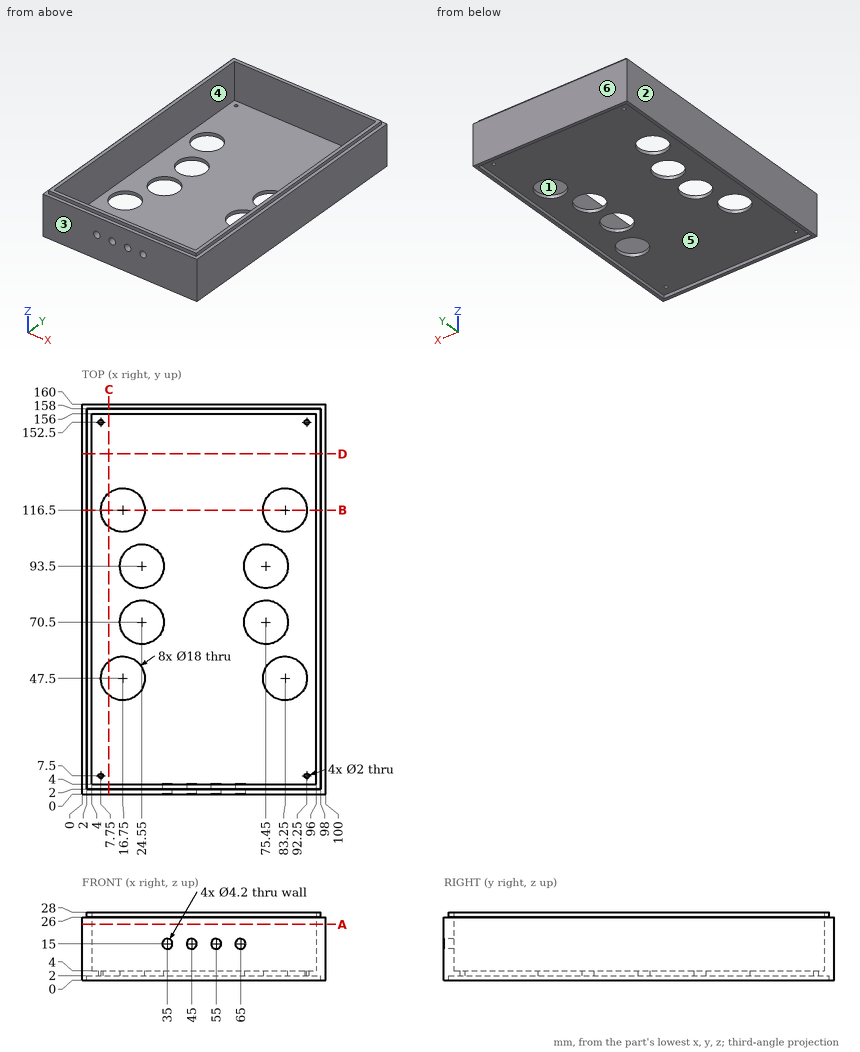
The figure shows three views and two pictorial views of one solid part (mm, origin at its lowest corner). Answer the questions. A direction names the side the tool comes from. Round coordinates to 2 decimals unless told otherwise and drop trailing zeros. Loops run counter-clockwise (first coordinate to the right, second up) from the corner with the lowest first, then second, coordinate; pieces in that order, holes last. Notation, with made-up numbers: M 0,76 L 4,76 A27 cw 4,103 Z; hole C -15.5,24 d4. An arc over 180 degrees is marked long. Write each question's results on one line, items separated by ' | '. Start each with the question number.
1) Find section C-C on x = 11. Write down the section's boundary in (y, z).
2) Which of the six approach directions +Z, -Z, +X, -X, +Y, -Y give full straight-line access (tool end or side, diameter ignored) to the marked faces 4, 5 and 6?
3) Find section D-D on y = 139.5. Write down the section's boundary in (x, z), plus the area to 3 significant figures.
4) Straight lines are drawn through the part: probe 1 along X at (y, z) = (152.5, 2.8); probe 2 along X at (y, z) = (70.5, 3.25); probe 3 along Y at (x, z) = (38, 4.75). For each, find the intervals that lie inside material, in ascending order.
5) Determine the mould class of the marked faces 1, 2 and 3 for opening direction X: pulls with the +X half, pulls with the -X half, needs draft (parallel to the pull), parting line crosses it, or undercut.
6) Each of these flat-tipped pins is pushed along its axis until it touches: pin 1 (1.2 mm diameter, centred on x = 92.25, y = 7.5, fed in from +Z); pin 2 (6 mm diameter, centred on x = 31, y = 51.5, fed in from -Z); pin 3 (5 mm diameter, centred on x = 34, y = 117.5, fed in from +Z); pin 4 (0.6 mm diameter, centred on x = 57, z = 27, fed in from +Y). Where does it stop, or does it pass through?
7) Find section B-B on y = 116.5. Write down the section's boundary in (x, z), plus the area to 3 significant figures.
8) Find section A-A on z = 23. Write down the section's boundary in (x, y), plus the area to 3 significant figures.
Final values:
1) outline: M 0,0 L 2,0 L 2,2 L 40.58,2 L 40.58,4 L 4,4 L 4,28 L 2,28 L 2,26 L 0,26 Z; M 54.42,2 L 109.58,2 L 109.58,4 L 54.42,4 Z; M 123.42,2 L 158,2 L 158,0 L 160,0 L 160,26 L 158,26 L 158,28 L 156,28 L 156,4 L 123.42,4 Z
2) face 4: +Z | face 5: -Z | face 6: +Z, -Z, +X, -X, +Y
3) outline: M 0,0 L 2,0 L 2,2 L 98,2 L 98,0 L 100,0 L 100,26 L 98,26 L 98,28 L 96,28 L 96,4 L 4,4 L 4,28 L 2,28 L 2,26 L 0,26 Z | area: 392 mm²
4) probe 1: 0 to 6.75, 8.75 to 91.25, 93.25 to 100 | probe 2: 0 to 15.55, 33.55 to 66.45, 84.45 to 100 | probe 3: 0 to 4, 156 to 160
5) face 1: undercut | face 2: pulls with the -X half | face 3: needs draft
6) pin 1: through | pin 2: z = 2 | pin 3: z = 4 | pin 4: y = 158
7) outline: M 0,0 L 2,0 L 2,2 L 7.75,2 L 7.75,4 L 4,4 L 4,28 L 2,28 L 2,26 L 0,26 Z; M 25.75,2 L 74.25,2 L 74.25,4 L 25.75,4 Z; M 92.25,2 L 98,2 L 98,0 L 100,0 L 100,26 L 98,26 L 98,28 L 96,28 L 96,4 L 92.25,4 Z | area: 320 mm²
8) outline: M 0,0 L 100,0 L 100,160 L 0,160 Z; hole M 4,4 L 96,4 L 96,156 L 4,156 Z | area: 2,020 mm²
